```python
from build123d import *

# Parameters (mm, degrees)
BOSS_EXTRUDE1_DEPTH = 10


with BuildPart() as part:
    # Sketch2 → Boss-Extrude1 (new body)
    with BuildSketch(Plane.XY):
        with BuildLine():
            Line((124.641341211, 54.579558825), (124.641341211, 65.576654529))
            ThreePointArc((124.641341211, 65.576654529), (123.303990774, 68.805304092), (120.075341211, 70.142654529))
            Line((120.075341211, 70.142654529), (51.212390107, 70.142654529))
            ThreePointArc((51.212390107, 70.142654529), (47.983740544, 68.805304092), (46.646390107, 65.576654529))
            Line((46.646390107, 65.576654529), (46.646390107, 54.579558825))
            Line((46.646390107, 54.579558825), (37.522288645, 54.579558825))
            add(Edge.make_bspline(
                [(37.522288645, 54.579558825), (21.959514644, 56.51337661), (11.293168946, 73.672446471), (9.333160981, 87.851570435)],
                knots=[0, 0, 0, 0, 1, 1, 1, 1], degree=3))
            add(Edge.make_bspline(
                [(9.333160981, 87.851570435), (4.816885024, 115.123208654), (16.148817178, 140.412638245)],
                knots=[0, 0, 0, 1, 1, 1], degree=2))
            add(Edge.make_bspline(
                [(16.148817178, 140.412638245), (27.405872479, 166.530361958), (34.0318253, 194.214132047)],
                knots=[0, 0, 0, 1, 1, 1], degree=2))
            add(Edge.make_bspline(
                [(34.0318253, 194.214132047), (38.922769668, 226.832256951), (31.295716129, 258.863919402)],
                knots=[0, 0, 0, 1, 1, 1], degree=2))
            add(Edge.make_bspline(
                [(31.295716129, 258.863919402), (24.342240472, 277.969027169), (37.522288645, 281.482204385)],
                knots=[0, 0, 0, 1, 1, 1], degree=2))
            Line((37.522288645, 281.482204385), (41.820716746, 281.182482064))
            Line((41.820716746, 281.182482064), (56.678211753, 274.911461444))
            Line((56.678211753, 274.911461444), (56.678211753, 250.94461401))
            ThreePointArc((56.678211753, 250.94461401), (59.130020887, 245.025423145), (65.049211753, 242.57361401))
            Line((65.049211753, 242.57361401), (104.457119811, 242.57361401))
            ThreePointArc((104.457119811, 242.57361401), (109.86830274, 244.050097173), (113.779669547, 248.070310218))
            Line((113.779669547, 248.070310218), (115.046074428, 250.359514609))
            add(Edge.make_bspline(
                [(115.046074428, 250.359514609), (130.641476409, 242.603233813), (147.862901343, 240.41980261)],
                knots=[0, 0, 0, 1, 1, 1], degree=2))
            add(Edge.make_bspline(
                [(147.862901343, 240.41980261), (195.584291202, 244.368436644), (200.178603281, 300.299783152)],
                knots=[0, 0, 0, 1, 1, 1], degree=2))
            add(Edge.make_bspline(
                [(200.178603281, 300.299783152), (203.787730837, 309.531782357), (209.479274597, 299.515490412)],
                knots=[0, 0, 0, 1, 1, 1], degree=2))
            add(Edge.make_bspline(
                [(209.479274597, 299.515490412), (220.319872334, 277.449577488), (214.75338425, 254.809889378)],
                knots=[0, 0, 0, 1, 1, 1], degree=2))
            add(Edge.make_bspline(
                [(214.75338425, 254.809889378), (211.622795841, 223.210356753), (186.430957093, 197.647557224), (191.264009323, 163.691313614)],
                knots=[0, 0, 0, 0, 1, 1, 1, 1], degree=3))
            add(Edge.make_bspline(
                [(191.264009323, 163.691313614), (196.854658148, 131.726086499), (212.699126926, 103.238239648)],
                knots=[0, 0, 0, 1, 1, 1], degree=2))
            add(Edge.make_bspline(
                [(212.699126926, 103.238239648), (228.353478754, 71.031768285), (236.75185914, 36.050820835)],
                knots=[0, 0, 0, 1, 1, 1], degree=2))
            add(Edge.make_bspline(
                [(236.75185914, 36.050820835), (238.174984629, 29.048757065), (237.427230612, 22.075105786)],
                knots=[0, 0, 0, 1, 1, 1], degree=2))
            add(Edge.make_bspline(
                [(237.427230612, 22.075105786), (229.298254036, 5.512025134), (213.990313769, 14.041488397)],
                knots=[0, 0, 0, 1, 1, 1], degree=2))
            add(Edge.make_bspline(
                [(213.990313769, 14.041488397), (194.666199965, 30.334432476), (174.369459856, 45.394945883)],
                knots=[0, 0, 0, 1, 1, 1], degree=2))
            add(Edge.make_bspline(
                [(174.369459856, 45.394945883), (159.806078551, 55.078070021), (141.198769972, 53.922244486), (124.641341211, 54.579558825)],
                knots=[0, 0, 0, 0, 1, 1, 1, 1], degree=3))
        make_face()
    extrude(amount=BOSS_EXTRUDE1_DEPTH)


solid = part.part
```
Design review of the part built by this model. Coordinates are the model's own, in mm. A direction names the side the tool comes from. Coordinates: 2 decimals unless noted, no trailing zeros. Order: outer loops, then holes, each group sorted by start corner. A loop starts at its lowest first (then second) coordinate and runs counter-clockwise, first axis right, second up. Notation, with made-up numbers: (-24, 59.5) -> (-14, 59.5) arc R11 cw to (-14, 63.5) -> close; hole circle Ø3 at (-29.5, 3). An arc over 180 degrees is marked (long way). One line per item, written item: value. Start each with the question number.
Q1. Tool access review of faces 1 (the flat face through (84, 242.574, 5)), 2 (the flat face through (123, 160, 0)), 3 (the flat face through (124.641, 60, 5)): name each direction out of +Z, -Z, +X, -X, +Y, -Y from which nothing blocks a thin tool from reaching the whole face with its end or side.
Q2. Insertion check: pin 1 Ø5 at (y, z) = (61, 6) entering from +X; pin 2 Ø1.5 at (y, z) = (98, 7) entering from +X; pin 3 Ø3 at (y, z) = (239, 6.5) entering from +X. Each pin has a flat end and moves straight along its axis. Give the tip position at first contact, or say it passes through.
Q3. Mouldability with a two-part tool opening along X and no side actions: class faces 4 (the flat face through (46.646, 60, 5)), 5 (the flat face through (42, 54.58, 5)) as pulls with the +X half, pulls with the -X half, needs draft (parallel to the pull), parting line crosses it, or undercut.
Q4. For probe 1 along X at (y, z) = (249.5, 1.75); probe 2 along X at (y, z) = (63.5, 9.5); probe 3 along X at (y, z) = (278.5, 1.5), list the stretches that pass through material, from the lowest coordinate up.
Q5. Take a section at A-A, the plane x = 107.5. State the section outline as (y, z) points.
Values follow:
1. face 1: +Z, -Z, +Y
1. face 2: -Z, +X, -X, +Y, -Y
1. face 3: +Z, -Z, -Y
2. pin 1: stops at x = 230.53
2. pin 2: stops at x = 215.54
2. pin 3: stops at x = 211.9
3. face 4: undercut
3. face 5: needs draft
4. probe 1: x = 33.26 to 56.8, 114.57 to 116.82, 175.91 to 214.02
4. probe 2: x = 21 to 46.65, 124.64 to 228.9
4. probe 3: x = 31.92 to 48.18, 196.16 to 216.07
5. outline: (70.14, 0) -> (243.02, 0) -> (243.02, 10) -> (70.14, 10) -> close
